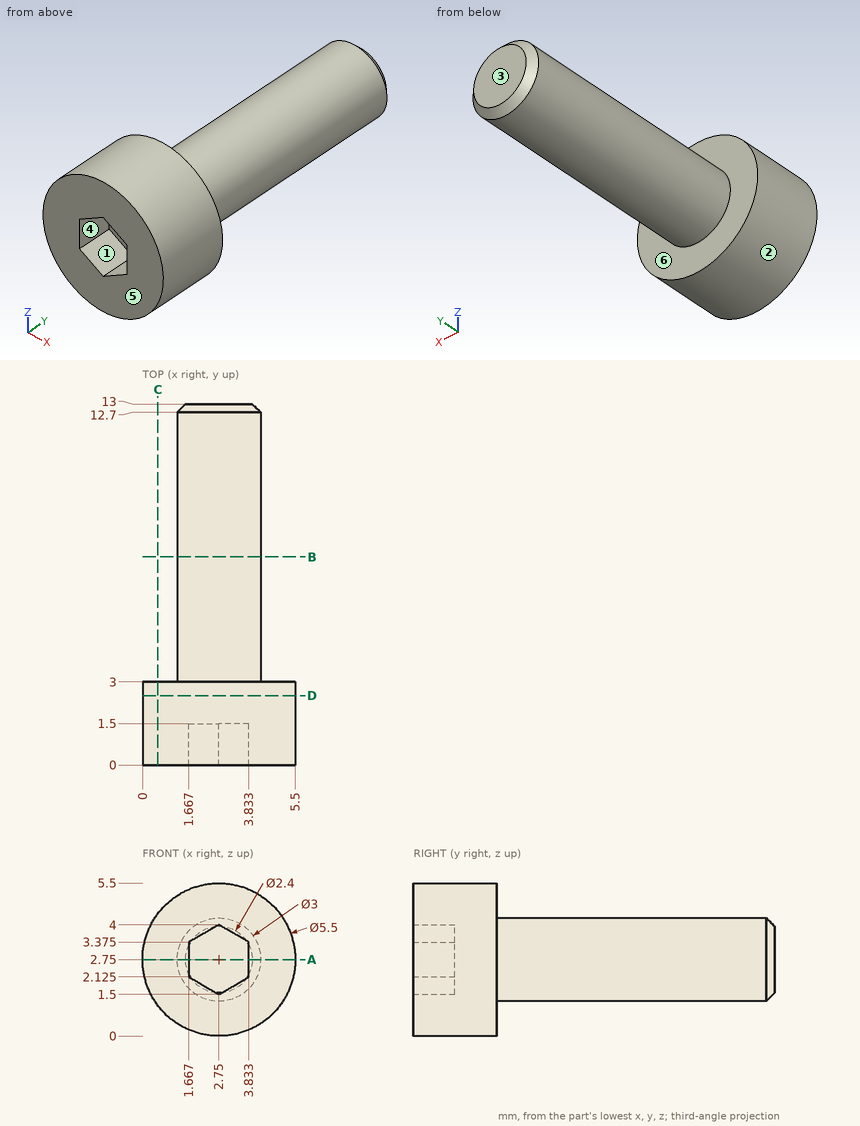
For this review, use the dimensioned drawing (mm, ordinates from the lowest corner) and the shaded views. A direction names the side the tool comes from. Give positions to 0.01 mm unless a question says otherwise; leave off trailing zeros. Loops run counter-clockwise (first coordinate to the right, second up) from the corner with the lowest first, then second, coordinate; pieces in that order, holes last. Notation, with made-up numbers: (-3.75, -20.75) - (38.25, -20.75) arc R23 ccw to (38.25, 3.25) - close; hole circle Ø1 at (21.25, 77.5). An arc over 180 degrees is marked (long way). Write each question's results on one line, items separated by ' | '.
(1) Take a section at A-A (z = 2.75). Give the boundary of the cut face in (x, y).
Conclusion:
outline: (0, 0) - (1.67, 0) - (1.67, 1.5) - (3.83, 1.5) - (3.83, 0) - (5.5, 0) - (5.5, 3) - (4.25, 3) - (4.25, 12.7) - (3.95, 13) - (1.55, 13) - (1.25, 12.7) - (1.25, 3) - (0, 3) - close
(2) For the marked faces 5 and 6, list the 3-axis set-ups (+Z, -Z, +X, -X, +Y, -Y) from which the entire face can be reached by the end or side of a thin tool; tool diameter is ignored.
Conclusion:
face 5: +Z, -Z, +X, -X, -Y | face 6: +Y
(3) For pin 1 Ø2 at (x, y) = (2, 11) entering from -Z, flat-tipped, find the tip position at first contact; note if it passes through.
Conclusion:
pin 1: z = 1.25
(4) For line 1 along Y through (x, z) = (1.35, 1.8); line 2 along Y through (x, z) = (3, 1.9); line 3 along X through (y, z) = (3.5, 2.5), list the stretches that pass through material, from the lowest coordinate up.
Conclusion:
line 1: 0 to 3 | line 2: 1.5 to 13 | line 3: 1.27 to 4.23
(5) Take a section at C-C (x = 0.55). Give the boundary of the cut face in (y, z).
Conclusion:
outline: (0, 1.1) - (3, 1.1) - (3, 4.4) - (0, 4.4) - close
(6) Draft analysis for pull direction Z (two halves, no side actions). For the marked faces 1, 2, 3 and 4, state which applies: +Z half, -Z half, draft (parallel to the pull), parting line (faces both ways), or undercut.
Conclusion:
face 1: undercut | face 2: parting line | face 3: draft | face 4: undercut
(7) Take a section at B-B (y = 7.5). Give the boundary of the cut face in (x, z).
Conclusion:
outline: circle Ø3 at (2.75, 2.75)
(8) Take a section at D-D (y = 2.5). Give the boundary of the cut face in (x, z).
Conclusion:
outline: circle Ø5.5 at (2.75, 2.75)
